Input: part model. Units: mm. Frame: model coordinates. A direction names the side the tool comes from. Coordinates: 2 decimals unless noted, no trailing zeros. Write each loop counter-clockwise with the first axis right and the second up, starting at its lowest first coordinate (ties: lowest second). Pieces come first, ordered by that corner, then holes. Notation, with made-up numbers: (22.25, -29.75) - (57.25, -29.75) arc R33 ccw to (57.25, 5.25) - close; hole circle Ø1 at (83.25, -36.75). An arc over 180 degrees is marked (long way). Use a Markdown table: item, result. Add a question column.
Q1. Material intervals for probe 1 along X at (y, z) = (4.25, -15); probe 2 along Z at (x, y) = (10, 31); probe 3 along Y at (x, z) = (8.5, -15.75), sorted ascending. Write a range as from..to.
Q2. Section query B-B (z = -2.75). Return the cut outline in (x, y).
Q3. Set-up query: faces 1 (the face through (70, 5, -15)), 2 (the face through (20, 29, -15)), 3 (the face through (35, 10, -12)). Return all of +Z, -Z, +X, -X, +Y, -Y with unobstructed straight access to the full face (end or side cutting, diameter ignored); none if empty.
Q4. Section query A-A (x = 60). Return the cut outline in (y, z).
Q5. Mould query, pull axis Z, two halves, no side actions, for faces 4 (the face through (14.77, 30.07, -11.5)), 5 (the face through (8, 25, -15)), 6 (the face through (15, 17, -20)). Classes: released by +Z, released by -Z, zero draft, split by the parting line, or undercut.
Q6. Pin query (flat end, axial travel): P1, Ø6, axis at x = 60, z = -15, coming from the +Y side; P2, Ø5, axis at x = 25, z = -25.5, coming from the +Y side; P3, Ø7.5, axis at y = 29, z = -9, coming from the +X side; P4, Ø9, axis at x = 10, z = -10, coming from the +Y side. Return the tip coordinate at first contact, or that it passes through.
Q7. Section query C-C (y = 9). Return the cut outline in (x, z).
Q8. Section query D-D (y = 27.5). Return the cut outline in (x, z).
from build123d import *

# Parameters (mm, degrees)
SKETCH1_W           = 70
SKETCH1_H           = 30
BOSS_EXTRUDE2_DEPTH = 10
SKETCH3_W           = 30
SKETCH3_H           = 10
BOSS_EXTRUDE3_DEPTH = 25
SKETCH4_W           = 10
SKETCH4_H           = 15
CUT_EXTRUDE1_DEPTH  = 11
SKETCH5_W           = 20
SKETCH5_H           = 10
BOSS_EXTRUDE4_DEPTH = 20
SKETCH6_R           = 5
CUT_EXTRUDE2_DEPTH  = 11
SKETCH7_R           = 5
CUT_EXTRUDE3_DEPTH  = 15


with BuildPart() as part:
    # Sketch1 → Boss-Extrude2 (new body)
    with BuildSketch(Plane(origin=(0, 0, 0), x_dir=(1, 0, 0), z_dir=(0, 1, 0))):
        with Locations((35, 15)):
            Rectangle(SKETCH1_W, SKETCH1_H)
    extrude(amount=BOSS_EXTRUDE2_DEPTH)

    # Sketch3 → Boss-Extrude3 (add)
    with BuildSketch(Plane(origin=(0, 10, 0), x_dir=(1, 0, 0), z_dir=(0, 1, 0))):
        with Locations((15, 25)):
            Rectangle(SKETCH3_W, SKETCH3_H)
    extrude(amount=BOSS_EXTRUDE3_DEPTH)

    # Sketch4 → Cut-Extrude1 (cut, through all)
    with BuildSketch(Plane.XY.offset(-20)):
        with Locations((25, 27.5)):
            Rectangle(SKETCH4_W, SKETCH4_H)
    extrude(amount=-CUT_EXTRUDE1_DEPTH, mode=Mode.SUBTRACT)

    # Sketch5 → Boss-Extrude4 (add)
    with BuildSketch(Plane.XY.offset(-20)):
        with Locations((10, 30)):
            Rectangle(SKETCH5_W, SKETCH5_H)
    extrude(amount=BOSS_EXTRUDE4_DEPTH)

    # Sketch6 → Cut-Extrude2 (cut, through all)
    with BuildSketch(Plane(origin=(0, 10, 0), x_dir=(1, 0, 0), z_dir=(0, 1, 0))):
        with Locations((40, 15)):
            Circle(SKETCH6_R)
        with Locations((60, 15)):
            Circle(SKETCH6_R)
    extrude(amount=-CUT_EXTRUDE2_DEPTH, mode=Mode.SUBTRACT)

    # Sketch7 → Cut-Extrude3 (cut)
    with BuildSketch(Plane(origin=(0, 35, 0), x_dir=(1, 0, 0), z_dir=(0, 1, 0))):
        with Locations((10, 10)):
            Circle(SKETCH7_R)
    extrude(amount=-CUT_EXTRUDE3_DEPTH, mode=Mode.SUBTRACT)


solid = part.part
Values follow:
| question | item | result |
|---|---|---|
| 1 | probe 1 | 0..35, 45..55, 65..70 |
| 1 | probe 2 | -30..-15, -5..0 |
| 1 | probe 3 | 0..10, 25..35 |
| 2 | outline | (0, 0) - (70, 0) - (70, 10) - (0, 10) - close; (0, 25) - (20, 25) - (20, 35) - (0, 35) - close |
| 3 | face 1 | +Z, -Z, +X, +Y, -Y |
| 3 | face 2 | +Z, -Z, +X, +Y |
| 3 | face 3 | +Z, +X |
| 4 | outline | (0, -30) - (10, -30) - (10, -20) - (0, -20) - close; (0, -10) - (10, -10) - (10, 0) - (0, 0) - close |
| 5 | face 4 | undercut |
| 5 | face 5 | zero draft |
| 5 | face 6 | released by +Z |
| 6 | P1 | through |
| 6 | P2 | y = 20 |
| 6 | P3 | x = 20 |
| 6 | P4 | y = 10 |
| 7 | outline | (0, -30) - (70, -30) - (70, 0) - (0, 0) - close; hole circle Ø10 at (40, -15); hole circle Ø10 at (60, -15) |
| 8 | outline | (0, -30) - (20, -30) - (20, 0) - (0, 0) - close; hole circle Ø10 at (10, -10) |
